Read the model definition and answer for the solid it produces. Units are mm, in the model's axes. A direction names the side the tool comes from. Round coordinates to 2 decimals unless told otherwise and drop trailing zeros. Loops run counter-clockwise (first coordinate to the right, second up) from the corner with the lowest first, then second, coordinate; pieces in that order, holes last. Notation, with made-up numbers: M -17,9.5 L 17,9.5 A23 ccw 17,19.5 Z; hole C 17,28 d10. An arc over 180 degrees is marked long. Write each question's results on one line, items separated by ' | '.
from build123d import *

# Parameters (mm, degrees)
SALIENTE_EXTRUIR1_DEPTH = 10
CROQUIS2_W              = 18
CROQUIS2_H              = 12.394708995
CORTAR_EXTRUIR1_DEPTH   = 5
REDONDEO1_R             = 3
REDONDEO2_R             = 3
REDONDEO3_R             = 1
CROQUIS3_R              = 3
CORTAR_EXTRUIR2_DEPTH   = 15


with BuildPart() as part:
    # Croquis1 → Saliente-Extruir1 (new body)
    with BuildSketch(Plane(origin=(0, 0, 0), x_dir=(0, 0, -1), z_dir=(1, 0, 0))):
        Polygon((0, -10.216508635), (0, 27.394708995), (-24, 27.394708995), (-24, 14.942424084), (-87.663818946, 14.942424084), (-87.663818946, -6.057575916), (-24, -6.057575916), (-24, -16.002849809), (0, -16.002849809), align=None)
    extrude(amount=SALIENTE_EXTRUIR1_DEPTH)

    # Croquis2 → Cortar-Extruir1 (cut)
    with BuildSketch(Plane(origin=(10, 0, 0), x_dir=(0, 0, -1), z_dir=(1, 0, 0))):
        with Locations((-9, 6.197354498)):
            Rectangle(CROQUIS2_W, CROQUIS2_H)
    extrude(amount=-CORTAR_EXTRUIR1_DEPTH, mode=Mode.SUBTRACT)

    # Redondeo1
    redondeo1_edges = [part.edges().sort_by_distance(p)[0] for p in [
        (5, -6.057575916, 24),
        (5, 14.942424084, 24),
    ]]
    fillet(redondeo1_edges, radius=REDONDEO1_R)

    # Redondeo2
    redondeo2_edges = [part.edges().sort_by_distance(p)[0] for p in [
        (5, -16.002849809, 24),
        (5, -6.057575916, 87.663818946),
        (5, 14.942424084, 87.663818946),
        (5, 27.394708995, 24),
    ]]
    fillet(redondeo2_edges, radius=REDONDEO2_R)

    # Redondeo3
    redondeo3_edges = [part.edges().sort_by_distance(p)[0] for p in [
        (7.5, 0, 18),
        (7.5, 12.394708995, 18),
    ]]
    fillet(redondeo3_edges, radius=REDONDEO3_R)

    # Croquis3 → Cortar-Extruir2 (cut)
    with BuildSketch(Plane(origin=(10, 0, 0), x_dir=(0, 0, -1), z_dir=(1, 0, 0))):
        with Locations((-79.963818946, 6.197354497)):
            Circle(CROQUIS3_R)
        with Locations((-72.263818946, 6.197354497)):
            Circle(CROQUIS3_R)
        with Locations((-64.563818946, 6.197354497)):
            Circle(CROQUIS3_R)
        with Locations((-56.863818946, 6.197354497)):
            Circle(CROQUIS3_R)
        with Locations((-49.163818946, 6.197354497)):
            Circle(CROQUIS3_R)
    extrude(amount=-CORTAR_EXTRUIR2_DEPTH, mode=Mode.SUBTRACT)


solid = part.part
Item 1: The part is cut by section D-D (z = 59). Determine the outline of the cut face in (x, y).
Outcome:
outline: M 0,-6.06 L 10,-6.06 L 10,4.09 L 0,4.09 Z; M 0,8.3 L 10,8.3 L 10,14.94 L 0,14.94 Z
Item 2: The part is cut by section C-C (x = 3.25). Determine the outline of the cut face in (y, z), plus the area to 3 significant figures.
Outcome:
outline: M -16,0 L 27.39,0 L 27.39,21 A3 ccw 24.39,24 L 17.94,24 A3 cw 14.94,27 L 14.94,84.66 A3 ccw 11.94,87.66 L -3.06,87.66 A3 ccw -6.06,84.66 L -6.06,27 A3 cw -9.06,24 L -13,24 A3 ccw -16,21 Z; hole C 6.2,49.16 d6; hole C 6.2,56.86 d6; hole C 6.2,64.56 d6; hole C 6.2,72.26 d6; hole C 6.2,79.96 d6 | area: 2,230 mm2
Item 3: Straight lines are drawn through the part: line 1 (Z direction, x = 1.5, y = 7); line 2 (Z direction, x = 4, y = 21); line 3 (Y direction, x = 9.5, z = 38). For each, find the intervals that lie inside material, in ascending order.
Outcome:
line 1: z = 0 to 46.27, 52.05 to 53.97, 59.75 to 61.67, 67.45 to 69.37, 75.15 to 77.07, 82.85 to 87.66 | line 2: z = 0 to 24 | line 3: y = -6.06 to 14.94
Item 4: The part is cut by section A-A (y = 4.5). Determine the outline of the cut face in (x, z), plus the area to 3 significant figures.
Outcome:
outline: M 0,0 L 5,0 L 5,18 L 10,18 L 10,46.69 L 0,46.69 Z; M 0,51.64 L 10,51.64 L 10,54.39 L 0,54.39 Z; M 0,59.34 L 10,59.34 L 10,62.09 L 0,62.09 Z; M 0,67.04 L 10,67.04 L 10,69.79 L 0,69.79 Z; M 0,74.74 L 10,74.74 L 10,77.49 L 0,77.49 Z; M 0,82.44 L 10,82.44 L 10,87.66 L 0,87.66 Z | area: 539 mm2
Item 5: Flat-ended cylindrical pins translate along their axes: pin 1 (3 mm diameter, centred on x = 3, y = -12, fed in from +Z); pin 2 (3 mm diameter, centred on x = 6.5, z = 45.5, fed in from +Y); pin 3 (1.5 mm diameter, centred on x = 8, y = 3.5, fed in from -Z); pin 4 (3.5 mm diameter, centred on y = 6.2, z = 72.26, fed in from +X). Find the tip coordinate at first contact, or state that the pin passes through.
Outcome:
pin 1: stops at z = 24 | pin 2: stops at y = 14.94 | pin 3: stops at z = 18 | pin 4: passes through
Item 6: The part is cut by section B-B (z = 16). Determine the outline of the cut face in (x, y), plus the area to 3 significant figures.
Outcome:
outline: M 0,-16 L 10,-16 L 10,0 L 5,0 L 5,12.39 L 10,12.39 L 10,27.39 L 0,27.39 Z | area: 372 mm2
Item 7: The mould has two halves that part along Y. Classify faces 1 (the face through (5.07, 7.098, 61.702)), 2 (the face through (10, 6, 35)), 3 (the face through (5, -6.058, 56)), 4 (the face through (5, 27.395, 10)): pulls with the +Y half, pulls with the -Y half, needs draft (parallel to the pull), parting line crosses it, or undercut.
Outcome:
face 1: undercut | face 2: needs draft | face 3: pulls with the -Y half | face 4: pulls with the +Y half
Item 8: For faces 5 (the face through (5, -11, 24)), 6 (the face through (8, 0, 9)), 7 (the face through (5, 21, 24)), 8 (the face through (5.07, 4.372, 82.345)), 9 (the face through (0, 6, 35)), determine the directions among +Z, -Z, +X, -X, +Y, -Y from which every point of the face is accessible in a straight line to the end or side of a thin tool.
Outcome:
face 5: +Z, +X, -X, -Y | face 6: -Z, +X | face 7: +Z, +X, -X, +Y | face 8: +X, -X | face 9: +Z, -Z, -X, +Y, -Y
